from build123d import *

# Parameters (mm, degrees)
SKETCH1_R           = 0.889
SKETCH1_R_2         = 1.1303
SKETCH1_W           = 6.35
SKETCH1_H           = 15.24
BOSS_EXTRUDE1_DEPTH = 6.35
SKETCH2_R           = 1.1684
CUT_EXTRUDE1_DEPTH  = 6.35


with BuildPart() as part:
    # Sketch1 → Boss-Extrude1 (new body)
    with BuildSketch(Plane(origin=(0, 0, 0), x_dir=(1, 0, 0), z_dir=(0, 1, 0))):
        with BuildLine():
            Line((-147.642205972, 18.314662121), (-147.642205972, -22.960337879))
            Line((-147.642205972, -22.960337879), (-122.242205972, -22.960337879))
            Line((-122.242205972, -22.960337879), (-122.242205972, -59.409337879))
            Line((-122.242205972, -59.409337879), (-157.167205972, -59.409337879))
            ThreePointArc((-157.167205972, -59.409337879), (-159.412270002, -60.339273849), (-160.342205972, -62.584337879))
            Line((-160.342205972, -62.584337879), (-160.342205972, -183.234337879))
            ThreePointArc((-160.342205972, -183.234337879), (-159.412270002, -185.479401909), (-157.167205972, -186.409337879))
            Line((-157.167205972, -186.409337879), (-62.292205972, -186.409337879))
            Line((-62.292205972, -186.409337879), (-62.292205972, 86.513662121))
            Line((-62.292205972, 86.513662121), (-87.692205972, 86.513662121))
            Line((-87.692205972, 86.513662121), (-87.692205972, 92.863662121))
            Line((-87.692205972, 92.863662121), (-138.492205972, 92.863662121))
            Line((-138.492205972, 92.863662121), (-138.492205972, 86.513662121))
            Line((-138.492205972, 86.513662121), (-144.842205972, 86.513662121))
            Line((-144.842205972, 86.513662121), (-144.842205972, 80.163662121))
            Line((-144.842205972, 80.163662121), (-138.492205972, 80.163662121))
            Line((-138.492205972, 80.163662121), (-138.492205972, 61.113662121))
            Line((-138.492205972, 61.113662121), (-144.842205972, 61.113662121))
            Line((-144.842205972, 61.113662121), (-144.842205972, 54.763662121))
            Line((-144.842205972, 54.763662121), (-122.242205972, 54.763662121))
            Line((-122.242205972, 54.763662121), (-122.242205972, 18.314662121))
            Line((-122.242205972, 18.314662121), (-147.642205972, 18.314662121))
        make_face()
        with Locations(Location((-118.749705972, -27.815337973, 0), (0, 0, 270))):
            Circle(SKETCH1_R, mode=Mode.SUBTRACT)
        with Locations(Location((-118.749705972, 12.919662091, 0), (0, 0, 270))):
            Circle(SKETCH1_R, mode=Mode.SUBTRACT)
        with Locations(Location((-110.264705924, 12.919662091, 0), (0, 0, 270))):
            Circle(SKETCH1_R, mode=Mode.SUBTRACT)
        with Locations(Location((-110.264705924, -27.815337973, 0), (0, 0, 270))):
            Circle(SKETCH1_R, mode=Mode.SUBTRACT)
        with Locations(Location((-118.749705972, 51.271162121, 0), (0, 0, 270))):
            Circle(SKETCH1_R_2, mode=Mode.SUBTRACT)
        with Locations(Location((-118.749705972, 24.397962121, 0), (0, 0, 270))):
            Circle(SKETCH1_R_2, mode=Mode.SUBTRACT)
        with Locations(Location((-88.701505972, 51.271162121, 0), (0, 0, 270))):
            Circle(SKETCH1_R_2, mode=Mode.SUBTRACT)
        with Locations(Location((-88.701505972, 24.397962121, 0), (0, 0, 270))):
            Circle(SKETCH1_R_2, mode=Mode.SUBTRACT)
        with Locations(Location((-99.792205972, 13.177162121, 0), (0, 0, 270))):
            Circle(SKETCH1_R_2, mode=Mode.SUBTRACT)
        with Locations(Location((-99.792205972, -17.822837879, 0), (0, 0, 270))):
            Circle(SKETCH1_R_2, mode=Mode.SUBTRACT)
        with Locations(Location((-83.247205972, -65.124337879, 0), (0, 0, 270))):
            Circle(SKETCH1_R_2, mode=Mode.SUBTRACT)
        with Locations(Location((-86.422205972, -131.164337879, 0), (0, 0, 270))):
            Circle(SKETCH1_R_2, mode=Mode.SUBTRACT)
        with Locations((-104.549705924, -2.322837879)):
            Rectangle(SKETCH1_W, SKETCH1_H, mode=Mode.SUBTRACT)
    boss_extrude1 = extrude(amount=BOSS_EXTRUDE1_DEPTH)

    # Sketch2 → Cut-Extrude1 (cut)
    with BuildSketch(Plane(origin=(0, 6.35, 0), x_dir=(1, 0, 0), z_dir=(0, 1, 0))):
        with Locations(Location((-141.292205972, 15.177162121, 0), (0, 0, 270))):
            Circle(SKETCH2_R)
        with Locations(Location((-141.292205972, -19.822837879, 0), (0, 0, 270))):
            Circle(SKETCH2_R)
    cut_extrude1 = extrude(amount=-CUT_EXTRUDE1_DEPTH, mode=Mode.SUBTRACT)

    # Mirror1: Boss-Extrude1, Cut-Extrude1 across plane
    add(boss_extrude1.mirror(Plane(origin=(-62.292205972, 6.35, -86.513662121), x_dir=(0, 0, 1), z_dir=(-1, 0, 0))))
    add(cut_extrude1.mirror(Plane(origin=(-62.292205972, 6.35, -86.513662121), x_dir=(0, 0, 1), z_dir=(-1, 0, 0))), mode=Mode.SUBTRACT)


solid = part.part
The listing builds one solid part. Answer for the finished solid, in the listing's coordinates (mm). A direction names the side the tool comes from. Coordinates: 2 decimals unless noted, no trailing zeros. Order: outer loops, then holes, each group sorted by start corner. A loop starts at its lowest first (then second) coordinate and runs counter-clockwise, first axis right, second up. Notation, with made-up numbers: (-29, 19.25) -> (-25, 19.25) arc R15 ccw to (-25, 46.25) -> close; hole circle Ø11 at (14.25, 77). An arc over 180 degrees is marked (long way). Answer in a Markdown table with one row per item. Add a question column.
Item 1: Find section A-A (z = 3.5). Write down the section's boundary in (x, y).
Item 2: Find section D-D (z = 43.5). Write down the section's boundary in (x, y).
Item 3: Find section B-B (x = 9.5). Write down the section's boundary in (y, z).
Item 4: Determine the mould class of faces 6 (the face through (-113, 3, -92.864)), 7 (the face through (-61, 3, 186.409)), 8 (the face through (-36.892, 3, -90)), 9 (the face through (10, 3, -18.315)) for opening direction Z: +Z half, -Z half, draft (parallel to the pull), parting line (faces both ways), or undercut.
Item 5: Find the intervals of material crossed by L1, parallel to Z at x = 5, y = 4.5; L2, parallel to Z at x = -88, y = 5; L3, parallel to X at y = 2.5, z = -39.5, in increasing order. Write a range as from..to.
Item 6: Which of the six approach directions +Z, -Z, +X, -X, +Y, -Y give full straight-line access (tool end or side, diameter ignored) to faces 1 (the face through (-23.21, 3, 2)), 2 (the face through (-61, 6.35, 45)), 3 (the face through (-138.492, 3, -71)), 4 (the face through (-2.342, 3, -37)), 5 (the face through (23.058, 3, 2))?
Item 7: Find section C-C (y = 3.5). State how many separate pieces and enclosed holes the cut face has, then the cut area to 3 significant figures.
Item 8: This flat-tipped pin is pushed along its axis until it touches: P1, Ø3, axis at y = 3.5, z = 4, coming from the -X side. Where does it stop, or does it pass through?
Result set:
| question | item | result |
|---|---|---|
| 1 | outline | (-147.64, 0) -> (-107.72, 0) -> (-107.72, 6.35) -> (-147.64, 6.35) -> close; (-101.37, 0) -> (-23.21, 0) -> (-23.21, 6.35) -> (-101.37, 6.35) -> close; (-16.86, 0) -> (23.06, 0) -> (23.06, 6.35) -> (-16.86, 6.35) -> close |
| 2 | outline | (-122.24, 0) -> (-2.34, 0) -> (-2.34, 6.35) -> (-122.24, 6.35) -> close |
| 3 | outline | (0, -92.86) -> (6.35, -92.86) -> (6.35, -54.76) -> (0, -54.76) -> close; (0, -18.31) -> (6.35, -18.31) -> (6.35, 22.96) -> (0, 22.96) -> close; (0, 59.41) -> (6.35, 59.41) -> (6.35, 186.41) -> (0, 186.41) -> close |
| 4 | face 6 | -Z half |
| 4 | face 7 | +Z half |
| 4 | face 8 | draft |
| 4 | face 9 | undercut |
| 5 | L1 | z = -92.86..-54.76, -18.31..22.96, 59.41..186.41 |
| 5 | L2 | z = -92.86..-52.16, -50.38..-25.28, -23.51..186.41 |
| 5 | L3 | x = -122.24..-2.34 |
| 6 | face 1 | +Y, -Y |
| 6 | face 2 | +Z, -Z, +X, -X, +Y |
| 6 | face 3 | -X, +Y, -Y |
| 6 | face 4 | +X, +Y, -Y |
| 6 | face 5 | -Z, +X, +Y, -Y |
| 7 | separate pieces | 1 |
| 7 | enclosed holes | 30 |
| 7 | area | 46,000 mm² |
| 8 | P1 | stops at x = -147.64 |
